Check sheet for the drawn part. Datum: minimum x, y, z corner. Units: mm. Round coordinates to 2 decimals unless told otherwise and drop trailing zeros. Order: outer loops, then holes, each group sorted by start corner. A loop starts at its lowest first (then second) coordinate and runs counter-clockwise, first axis right, second up. Notation, with made-up numbers: (42, -21) -> (96, -21) arc R22 ccw to (96, -1) -> close; hole circle Ø7 at (56, 48). An arc over 180 degrees is marked (long way). Answer as CSV lines item,"result". Start each with the question number.
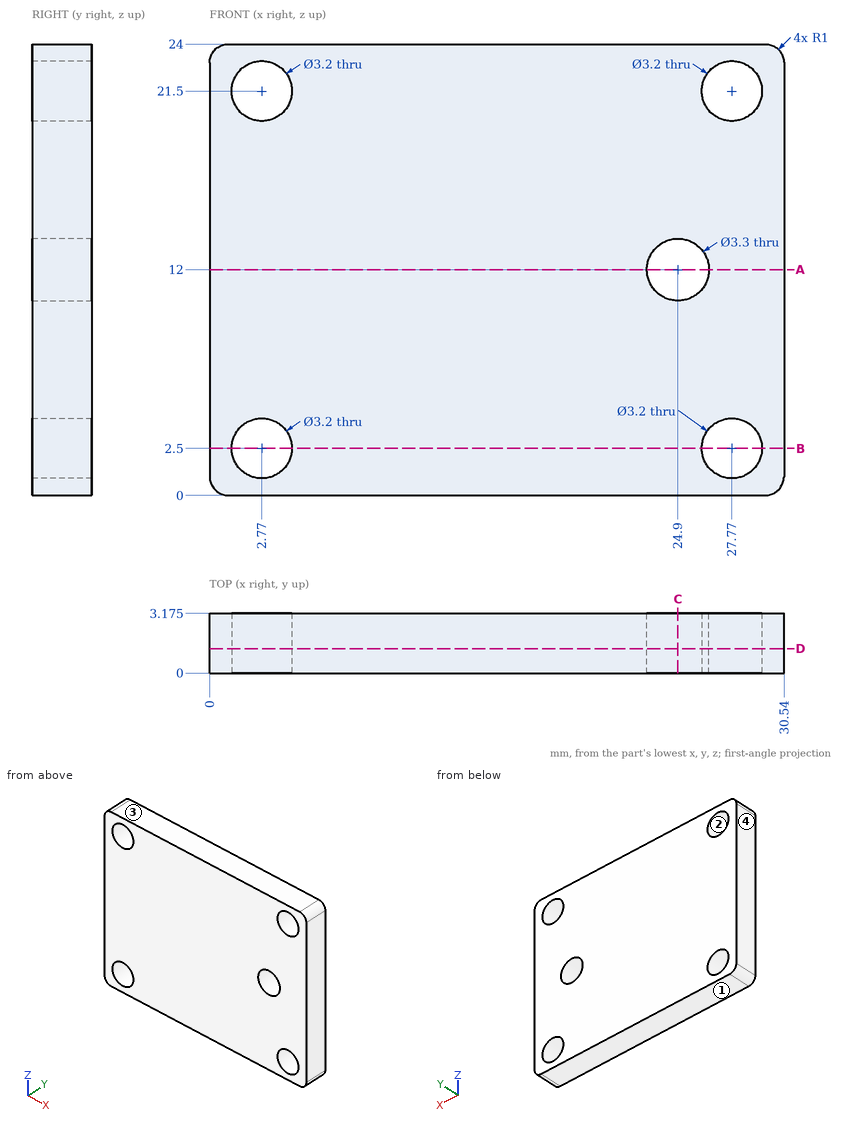
1) Mould release check, pull along Z, two halves, no side actions. Record for the marked faces 1, 2, 3 and 4: released by +Z, released by -Z, zero draft, split by the parting line, or undercut.
2) Depth check by flat-ended pin: pin 1 Ø8 at (x, z) = (7, 19.5) entering from -Y. Enter the tip coordinate at first touch or a pass-through.
3) Material ranges on line 1 along X through (y, z) = (2.05, 2.5); line 2 along Z through (x, y) = (27, 0.95); line 3 along X through (y, z) = (1.45, 3), recorded low to high.
4) Section check A-A on z = 12. Record the cut outline in (x, y) (3 decimals).
5) Section check C-C on x = 24.9. Record the cut outline in (y, z) (3 decimals), then the cut area to 3 significant figures.
6) Section check D-D on y = 1.3. Record the cut outline in (x, z), then the cut area to 3 significant figures.
7) Section check B-B on z = 2.5. Record the cut outline in (x, y) (3 decimals).
Solutions:
1,face 1,"released by -Z"
1,face 2,"undercut"
1,face 3,"released by +Z"
1,face 4,"zero draft"
2,pin 1,"stops at y = 0"
3,line 1,"x = 0 to 1.17, 4.37 to 26.17, 29.37 to 30.54"
3,line 2,"z = 0 to 1.1, 3.9 to 20.1, 22.9 to 24"
3,line 3,"x = 0 to 1.25, 4.29 to 26.25, 29.29 to 30.54"
4,outline,"(0, 0) -> (23.25, 0) -> (23.25, 3.175) -> (0, 3.175) -> close; (26.55, 0) -> (30.54, 0) -> (30.54, 3.175) -> (26.55, 3.175) -> close"
5,outline,"(0, 0) -> (3.175, 0) -> (3.175, 10.35) -> (0, 10.35) -> close; (0, 13.65) -> (3.175, 13.65) -> (3.175, 24) -> (0, 24) -> close"
5,area,"65.7 mm^2"
6,outline,"(0, 1) arc R1 ccw to (1, 0) -> (29.54, 0) arc R1 ccw to (30.54, 1) -> (30.54, 23) arc R1 ccw to (29.54, 24) -> (1, 24) arc R1 ccw to (0, 23) -> close; hole circle Ø3.2 at (2.77, 2.5); hole circle Ø3.2 at (2.77, 21.5); hole circle Ø3.3 at (24.9, 12); hole circle Ø3.2 at (27.77, 2.5); hole circle Ø3.2 at (27.77, 21.5)"
6,area,"691 mm^2"
7,outline,"(0, 0) -> (1.17, 0) -> (1.17, 3.175) -> (0, 3.175) -> close; (4.37, 0) -> (26.17, 0) -> (26.17, 3.175) -> (4.37, 3.175) -> close; (29.37, 0) -> (30.54, 0) -> (30.54, 3.175) -> (29.37, 3.175) -> close"
